from build123d import *
from build123d.topology import SkipClean

# Parameters (mm, degrees)
SKETCH1_W           = 38.06
SKETCH1_H           = 10.25
BOSS_EXTRUDE1_DEPTH = 0.6
SKETCH2_R           = 1.65
CUT_EXTRUDE1_DEPTH  = 0.6
SKETCH3_W           = 17.88
SKETCH3_H           = 0.6
BOSS_EXTRUDE2_DEPTH = 5.01
BOSS_EXTRUDE3_DEPTH = 17.88
CUT_EXTRUDE2_DEPTH  = 17.88


with BuildPart() as part:
    # Sketch1 → Boss-Extrude1 (new body)
    with BuildSketch(Plane.XY):
        with Locations((19.03, -5.125)):
            Rectangle(SKETCH1_W, SKETCH1_H)
    extrude(amount=BOSS_EXTRUDE1_DEPTH)

    # Sketch2 → Cut-Extrude1 (cut)
    with BuildSketch(Plane.XY.offset(0.6)):
        with Locations((4.93, -4.62)):
            Circle(SKETCH2_R)
        with Locations((33.13, -4.62)):
            Circle(SKETCH2_R)
    extrude(amount=-CUT_EXTRUDE1_DEPTH, mode=Mode.SUBTRACT)

    # Sketch3 → Boss-Extrude2 (add)
    with BuildSketch(Plane.XZ.offset(10.25)):
        with Locations((19.03, 0.3)):
            Rectangle(SKETCH3_W, SKETCH3_H)
    extrude(amount=BOSS_EXTRUDE2_DEPTH)

    # Sketch4 → Boss-Extrude3 (add)
    with BuildSketch(Plane(origin=(27.97, 0, 0), x_dir=(0, 0, -1), z_dir=(1, 0, 0))):
        with BuildLine():
            Line((-2, -11.86), (-2, -11.26))
            ThreePointArc((-2, -11.26), (-3.414213562, -14.674213562), (0, -13.26))
            Line((0, -13.26), (-0.6, -13.26))
            ThreePointArc((-0.6, -13.26), (-2.989949494, -14.249949494), (-2, -11.86))
        make_face()
    extrude(amount=-BOSS_EXTRUDE3_DEPTH)

    # Sketch5 → Cut-Extrude2 (cut)
    with SkipClean():  # the faces are left unmerged after this step: merging them gives an invalid solid
        with BuildSketch(Plane(origin=(27.97, 0, 0), x_dir=(0, 0, -1), z_dir=(1, 0, 0))):
            with BuildLine():
                ThreePointArc((0, -13.26), (-0.156091109, -14.034596669), (-0.6, -14.688285686))
                Line((-0.6, -14.688285686), (-0.6, -15.26))
                Line((-0.6, -15.26), (0, -15.26))
                Line((0, -15.26), (0, -13.26))
            make_face()
        extrude(amount=-CUT_EXTRUDE2_DEPTH, mode=Mode.SUBTRACT)


solid = part.part
Verification items for the finished model (mm, model axes). A direction names the side the tool comes from. Coordinates: 2 decimals unless noted, no trailing zeros. Write each loop counter-clockwise with the first axis right and the second up, starting at its lowest first coordinate (ties: lowest second). Pieces come first, ordered by that corner, then holes. Notation, with made-up numbers: (66, 62) -> (85, 62) arc R30 ccw to (85, 90) -> close; hole circle Ø10 at (61.5, 36.5). An arc over 180 degrees is marked (long way). One line per item, written item: value. Start each with the question number.
Q1. Thickness scan on L1, parallel to Y at x = 4.93, z = 0.15; L2, parallel to Z at x = 24, y = -13.26; L3, parallel to X at y = -3.5, z = 0.5. Record the ranges inside material, lowest first. Write a range as from..to.
Q2. Mould release check, pull along Y, two halves, no side actions. Record for faces 4 (the cylindrical face through (31.914, -3.505, 0.304)), 5 (the flat face through (19, -7, 0.6)): pulls with the +Y half, pulls with the -Y half, needs draft (parallel to the pull), parting line crosses it, or undercut.
Q3. Cross-section at B-B on y = -4.62. Enter the section's corners in (x, z), and give its area (3 significant figures).
Q4. Go/stop test with flat-tipped pins: P1, Ø2, axis at x = 33.13, y = -4.62, coming from the +Z side; P2, Ø2, axis at y = -12.5, z = 3, coming from the -X side; P3, Ø1.2, axis at y = -12.5, z = 2.5, coming from the +X side; P4, Ø0.5, axis at x = 6, z = 0.5, coming from the -Y side. Record where each tip stops, or that it passes through.
Q5. Cross-section at A-A on x = 4.93. Enter the section's corners in (y, z), and give its area (3 significant figures).
Q6. Access from +Z, -Z, +X, -X, +Y, -Y to the whole of each face (thin tool, end or side, straight path). Record for faces 1 (the flat face through (19, -7, 0)), 2 (the flat face through (27.97, -13.7, 0.5)), 3 (the flat face through (10.09, -13.7, 0.5)).
Q7. Cross-section at D-D on y = -13.75. Enter the section's corners in (x, z), and give its area (3 significant figures).
Q8. Cross-section at C-C on x = 24. Enter the section's corners in (y, z), and give its area (3 significant figures).
Checked values:
1. L1: y = -10.25..-6.27, -2.97..0
1. L2: z = 0..0.6, 3.4..4
1. L3: x = 0..3.72, 6.14..31.92, 34.34..38.06
2. face 4: undercut
2. face 5: needs draft
3. outline: (0, 0) -> (3.28, 0) -> (3.28, 0.6) -> (0, 0.6) -> close; (6.58, 0) -> (31.48, 0) -> (31.48, 0.6) -> (6.58, 0.6) -> close; (34.78, 0) -> (38.06, 0) -> (38.06, 0.6) -> (34.78, 0.6) -> close
3. area: 18.9 mm²
4. P1: passes through
4. P2: stops at x = 10.09
4. P3: stops at x = 27.97
4. P4: stops at y = -10.25
5. outline: (-10.25, 0) -> (-6.27, 0) -> (-6.27, 0.6) -> (-10.25, 0.6) -> close; (-2.97, 0) -> (0, 0) -> (0, 0.6) -> (-2.97, 0.6) -> close
5. area: 4.17 mm²
6. face 1: -Z, +X, -X, +Y, -Y
6. face 2: +Z, -Z, +X, -Y
6. face 3: +Z, -Z, -X, -Y
7. outline: (10.09, 0.06) -> (27.97, 0.06) -> (27.97, 0.69) -> (10.09, 0.69) -> close; (10.09, 3.31) -> (27.97, 3.31) -> (27.97, 3.94) -> (10.09, 3.94) -> close
7. area: 22.4 mm²
8. outline: (-13.26, 0) -> (0, 0) -> (0, 0.6) -> (-13.26, 0.6) arc R1.4 cw (long way) to (-11.86, 2) -> (-11.26, 2) arc R2 ccw (long way) to start
8. area: 12.8 mm²
